```python
from build123d import *

# Parameters (mm, degrees)
SKETCH1_W               = 95
SKETCH1_H               = 75
BOSS_EXTRUDE1_DEPTH     = 5
BOSS_EXTRUDE4_DEPTH     = 45
SKETCH5_R               = 1.6
CUT_EXTRUDE1_DEPTH      = 91
CUT_EXTRUDE1_DEPTH_BACK = 6
CUT_EXTRUDE2_REACH      = 7
SKETCH6_R               = 1.6
BOSS_EXTRUDE5_DEPTH     = 5
BOSS_EXTRUDE6_START     = -90
BOSS_EXTRUDE6_DEPTH     = 5
CUT_EXTRUDE3_REACH      = 77
SKETCH8_R               = 1.6
CUT_EXTRUDE4_START      = -1.25
CUT_EXTRUDE4_DEPTH      = 2.5


with BuildPart() as part:
    # Sketch1 → Boss-Extrude1 (new body)
    with BuildSketch(Plane(origin=(0, 0, 0), x_dir=(1, 0, 0), z_dir=(0, 1, 0))):
        Rectangle(SKETCH1_W, SKETCH1_H)
    extrude(amount=BOSS_EXTRUDE1_DEPTH)

    # Sketch4 → Boss-Extrude4 (add)
    with BuildSketch(Plane(origin=(0, 5, 0), x_dir=(1, 0, 0), z_dir=(0, 1, 0))):
        Polygon((-47.5, 37.5), (-42.5, 37.5), (42.5, 37.5), (47.5, 37.5), (47.5, 12.5), (42.5, 12.5), (42.5, 32.5), (-42.5, 32.5), (-42.5, 12.5), (-47.5, 12.5), align=None)
    extrude(amount=BOSS_EXTRUDE4_DEPTH)

    # Sketch5 → Cut-Extrude1 (cut, two sides)
    with BuildSketch(Plane(origin=(-42.5, 0, 0), x_dir=(0, 0, -1), z_dir=(1, 0, 0))) as cut_extrude1_sk:
        with Locations((22.5, 35)):
            Circle(SKETCH5_R)
        with Locations((22.5, 20)):
            Circle(SKETCH5_R)
    extrude(amount=CUT_EXTRUDE1_DEPTH, mode=Mode.SUBTRACT)
    extrude(cut_extrude1_sk.sketch, amount=-CUT_EXTRUDE1_DEPTH_BACK, mode=Mode.SUBTRACT)

    # Sketch6 → Cut-Extrude2 (cut, up to next)
    with BuildSketch(Plane.XY.offset(-32.5), mode=Mode.PRIVATE) as cut_extrude2_sk1:
        with Locations((-32.5, 35)):
            Circle(SKETCH6_R)
    cut_extrude2_tool1 = extrude(cut_extrude2_sk1.sketch, amount=-CUT_EXTRUDE2_REACH, mode=Mode.PRIVATE) & part.part
    add(cut_extrude2_tool1.solids().sort_by_distance((-32.5, 35, -32.5))[0], mode=Mode.SUBTRACT)
    # Sketch6 → Cut-Extrude2 (cut, up to next)
    with BuildSketch(Plane.XY.offset(-32.5), mode=Mode.PRIVATE) as cut_extrude2_sk2:
        with Locations((-32.5, 20)):
            Circle(SKETCH6_R)
    cut_extrude2_tool2 = extrude(cut_extrude2_sk2.sketch, amount=-CUT_EXTRUDE2_REACH, mode=Mode.PRIVATE) & part.part
    add(cut_extrude2_tool2.solids().sort_by_distance((-32.5, 20, -32.5))[0], mode=Mode.SUBTRACT)
    # Sketch6 → Cut-Extrude2 (cut, up to next)
    with BuildSketch(Plane.XY.offset(-32.5), mode=Mode.PRIVATE) as cut_extrude2_sk3:
        with Locations((32.5, 20)):
            Circle(SKETCH6_R)
    cut_extrude2_tool3 = extrude(cut_extrude2_sk3.sketch, amount=-CUT_EXTRUDE2_REACH, mode=Mode.PRIVATE) & part.part
    add(cut_extrude2_tool3.solids().sort_by_distance((32.5, 20, -32.5))[0], mode=Mode.SUBTRACT)
    # Sketch6 → Cut-Extrude2 (cut, up to next)
    with BuildSketch(Plane.XY.offset(-32.5), mode=Mode.PRIVATE) as cut_extrude2_sk4:
        with Locations((32.5, 35)):
            Circle(SKETCH6_R)
    cut_extrude2_tool4 = extrude(cut_extrude2_sk4.sketch, amount=-CUT_EXTRUDE2_REACH, mode=Mode.PRIVATE) & part.part
    add(cut_extrude2_tool4.solids().sort_by_distance((32.5, 35, -32.5))[0], mode=Mode.SUBTRACT)

    # Sketch7 → Boss-Extrude5 (add)
    with BuildSketch(Plane.ZY.offset(47.5)):
        Polygon((-12.5, 5), (-2.5, 5), (-12.5, 20), align=None)
    extrude(amount=-BOSS_EXTRUDE5_DEPTH)

    # Sketch7<2> → Boss-Extrude6 (add)
    with BuildSketch(Plane.ZY.offset(47.5).offset(BOSS_EXTRUDE6_START)):
        Polygon((-12.5, 5), (-2.5, 5), (-12.5, 20), align=None)
    extrude(amount=-BOSS_EXTRUDE6_DEPTH)

    # Sketch8 → Cut-Extrude3 (cut, up to next)
    with BuildSketch(Plane(origin=(0, 0, -37.5), x_dir=(-1, 0, 0), z_dir=(0, 0, -1)), mode=Mode.PRIVATE) as cut_extrude3_sk1:
        with Locations((-7.5, 35)):
            Circle(SKETCH8_R)
    cut_extrude3_tool1 = extrude(cut_extrude3_sk1.sketch, amount=-CUT_EXTRUDE3_REACH, mode=Mode.PRIVATE) & part.part
    add(cut_extrude3_tool1.solids().sort_by_distance((7.5, 35, -37.5))[0], mode=Mode.SUBTRACT)
    # Sketch8 → Cut-Extrude3 (cut, up to next)
    with BuildSketch(Plane(origin=(0, 0, -37.5), x_dir=(-1, 0, 0), z_dir=(0, 0, -1)), mode=Mode.PRIVATE) as cut_extrude3_sk2:
        with Locations((7.5, 35)):
            Circle(SKETCH8_R)
    cut_extrude3_tool2 = extrude(cut_extrude3_sk2.sketch, amount=-CUT_EXTRUDE3_REACH, mode=Mode.PRIVATE) & part.part
    add(cut_extrude3_tool2.solids().sort_by_distance((-7.5, 35, -37.5))[0], mode=Mode.SUBTRACT)

    # Sketch9 → Cut-Extrude4 (cut)
    with BuildSketch(Plane(origin=(0, 0, -37.5), x_dir=(-1, 0, 0), z_dir=(0, 0, -1)).offset(CUT_EXTRUDE4_START)):
        Polygon((-32.5, 38.435234102), (-35.475, 36.717617051), (-35.475, 33.282382949), (-32.5, 31.564765898), (-29.525, 33.282382949), (-29.525, 36.717617051), align=None)
        Polygon((-7.5, 38.435234102), (-10.475, 36.717617051), (-10.475, 33.282382949), (-7.5, 31.564765898), (-4.525, 33.282382949), (-4.525, 36.717617051), align=None)
        Polygon((7.5, 38.435234102), (4.525, 36.717617051), (4.525, 33.282382949), (7.5, 31.564765898), (10.475, 33.282382949), (10.475, 36.717617051), align=None)
        Polygon((32.5, 38.435234102), (29.525, 36.717617051), (29.525, 33.282382949), (32.5, 31.564765898), (35.475, 33.282382949), (35.475, 36.717617051), align=None)
        Polygon((32.5, 23.435234102), (29.525, 21.717617051), (29.525, 18.282382949), (32.5, 16.564765898), (35.475, 18.282382949), (35.475, 21.717617051), align=None)
        Polygon((-32.5, 23.435234102), (-35.475, 21.717617051), (-35.475, 18.282382949), (-32.5, 16.564765898), (-29.525, 18.282382949), (-29.525, 21.717617051), align=None)
    extrude(amount=-CUT_EXTRUDE4_DEPTH, mode=Mode.SUBTRACT)


solid = part.part
```
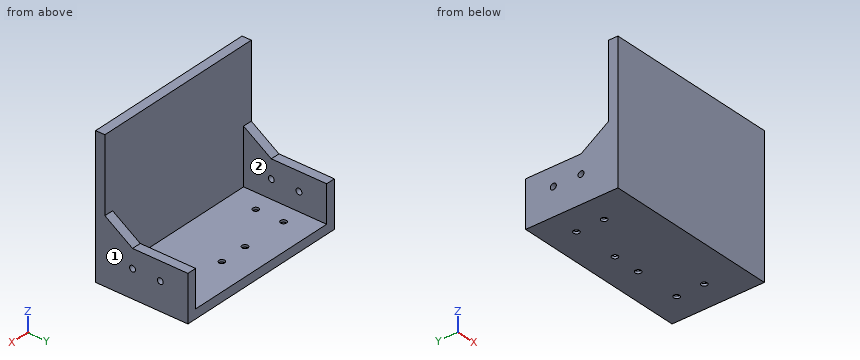
Read the model definition and answer for the solid it produces. Units are mm, in the model's axes. Face numbers are marked on the shaded views. A direction names the side the tool comes from. Give positions to 0.01 mm unless a question says otherwise; leave off trailing zeros. Write each loop counter-clockwise with the first axis right and the second up, starting at its lowest first coordinate (ties: lowest second). Pieces come first, ordered by that corner, then holes. Notation, with made-up numbers: (87.5, -27.5) -> (111.5, -27.5) arc R32 cw to (111.5, -1.5) -> close; hole circle Ø3 at (-36, -38.75). An arc over 180 degrees is marked (long way). Answer in a Markdown table with one row per item.
1) A tool of negligible diameter and unlimited length cuts with its end or side. For the marked faces 1 and 2, from which of +Z, -Z, +X, -X, +Y, -Y can it reach the whole face along a straight path? Write none if from no direction.
Results list:
| item | result |
|---|---|
| face 1 | +Z, -Z, +X, +Y, -Y |
| face 2 | +Z, +Y |
2) Straight lines are drawn through the part: line 1 (Y direction, x = 46.35, z = -22.5); line 2 (X direction, y = 47, z = -29.5); line 3 (Y direction, x = 32, z = -37). For each, find the intervals that lie inside material, in ascending order. Write a range as [from, to].
Results list:
| item | result |
|---|---|
| line 1 | [0, 18.4], [21.6, 33.4], [36.6, 50] |
| line 2 | [-47.5, -42.5], [42.5, 47.5] |
| line 3 | [0, 18.48], [21.52, 33.48], [36.52, 50] |
3) Section B-B on y = 35 is taken. Count the separate pieces of the cut face and the enclosed holes in it, plus the area to 4 significant figures.
Results list:
| item | result |
|---|---|
| separate pieces | 7 |
| enclosed holes | 0 |
| area | 551.5 mm^2 |
4) Each of these flat-tipped pins is pushed along its axis until it touches: pin 1 Ø1.8 at (x, y) = (-33.5, 34.5) entering from +Z; pin 2 Ø3 at (x, z) = (-0.5, -8.5) entering from +Y; pin 3 Ø1.9 at (x, y) = (-7.5, 35) entering from +Z. Where does it stop, or does it pass through?
Results list:
| item | result |
|---|---|
| pin 1 | z = -32.5 |
| pin 2 | y = 5 |
| pin 3 | through |
5) Section D-D on x = -22 is taken. Give the vertices of the cut face in (y, z).
Results list:
| item | result |
|---|---|
| outline | (0, -37.5) -> (50, -37.5) -> (50, -32.5) -> (5, -32.5) -> (5, 37.5) -> (0, 37.5) -> close |
6) Section A-A on z = -22.5 is taken. Give the vertices of the cut face in (x, y).
Results list:
| item | result |
|---|---|
| outline | (-47.5, 0) -> (47.5, 0) -> (47.5, 18.4) -> (42.5, 18.4) -> (42.5, 5) -> (-42.5, 5) -> (-42.5, 18.4) -> (-47.5, 18.4) -> close; (-47.5, 21.6) -> (-42.5, 21.6) -> (-42.5, 33.4) -> (-47.5, 33.4) -> close; (-47.5, 36.6) -> (-42.5, 36.6) -> (-42.5, 50) -> (-47.5, 50) -> close; (42.5, 21.6) -> (47.5, 21.6) -> (47.5, 33.4) -> (42.5, 33.4) -> close; (42.5, 36.6) -> (47.5, 36.6) -> (47.5, 50) -> (42.5, 50) -> close |
7) Section C-C on z = -31 is taken. Give the vertices of the cut face in (x, y).
Results list:
| item | result |
|---|---|
| outline | (-47.5, 0) -> (47.5, 0) -> (47.5, 50) -> (42.5, 50) -> (42.5, 5) -> (-42.5, 5) -> (-42.5, 50) -> (-47.5, 50) -> close |
